Design review of the part built by this model. Coordinates are the model's own, in mm. A direction names the side the tool comes from. Coordinates: 2 decimals unless noted, no trailing zeros. Write each loop counter-clockwise with the first axis right and the second up, starting at its lowest first coordinate (ties: lowest second). Pieces come first, ordered by that corner, then holes.
Q1. To check wall thickness, follow probe 1 along Z at (x, y) = (17, 17); probe 2 along Y at (x, z) = (93.5, 8.5); probe 3 along Y at (x, z) = (9.5, 7). State the ranges of each line that lie inside material, in increasing order.
Q2. Add section B-B, the plane x = 29. Give the boundary of the cut face in (y, z).
Q3. The part is to be moulded in two halves that separate along Z. For faces 4 (the face through (49, 20.802, 8)), 5 (the face through (50.7, -7.28, 16.28)), 6 (the face through (50.65, -9.83, 13.26)), 7 (the face through (50.651, 15.738, 7.519)), say which applies: +Z half, -Z half, draft (parallel to the pull), parting line (faces both ways), or undercut.
Q4. Machinability: for faces 1 (the face through (49, 19, 10.229)), 2 (the face through (98, -7, 15.073)), 3 (the face through (2, -7, 15.073)), which of the approach directions +Z, -Z, +X, -X, +Y, -Y give a long, thin tool a straight path to every point of the face, cutting with its end or side? Answer none if there is none.
Q5. Clearance check with flat-ended pins moving along their axes: pin 1 Ø8 at (y, z) = (0.5, 9) entering from -X; pin 2 Ø4 at (y, z) = (16.8, 8.07) entering from +X; pin 3 Ø2 at (x, z) = (34.5, 18) entering from +Y; pin 4 Ø5 at (y, z) = (-5.5, 18.5) entering from -X. State where each tip first meets the part, or that it passes through.
Q6. Add section A-A, the plane y = 19.5. Give the boundary of the cut face in (x, z).
Q7. Add section C-C, the plane z = 18.5. Give the boundary of the cut face in (x, y).
from build123d import *

# Parameters (mm, degrees)
SKETCH1_W           = 14
SKETCH1_H           = 27
BOSS_EXTRUDE1_DEPTH = 100
CUT_EXTRUDE1_DEPTH  = 100
FILLET1_R           = 10
SKETCH4_W           = 98.852101938
SKETCH4_H           = 4.155908349
BOSS_EXTRUDE2_DEPTH = 4
SKETCH5_R           = 1.2
SKETCH5_R_2         = 0.6
CUT_EXTRUDE2_DEPTH  = 100
CHAMFER1_SIZE       = 7
SKETCH6_W           = 4.155908349
SKETCH6_H           = 24
CUT_EXTRUDE3_DEPTH  = 3.5
SKETCH8_W           = 1.147898062
SKETCH8_H           = 4.155908349
BOSS_EXTRUDE3_DEPTH = 4
SKETCH9_W           = 4.155908349
SKETCH9_H           = 24
CUT_EXTRUDE4_DEPTH  = 3.5
SKETCH10_W          = 10.233519384
SKETCH10_H          = 31.339386183
CUT_EXTRUDE5_DEPTH  = 3.5
SKETCH11_W          = 18.924548437
SKETCH11_H          = 36.127134787
CUT_EXTRUDE7_DEPTH  = 3.5
FILLET2_R           = 5
FILLET5_R           = 1
FILLET6_R           = 1


with BuildPart() as part:
    # Sketch1 → Boss-Extrude1 (new body)
    with BuildSketch(Plane(origin=(0, 0, 0), x_dir=(0, 0, -1), z_dir=(1, 0, 0))):
        with Locations((-13.07263952, 3.302202671)):
            Rectangle(SKETCH1_W, SKETCH1_H)
    extrude(amount=BOSS_EXTRUDE1_DEPTH)

    # Sketch2 → Cut-Extrude1 (cut)
    with BuildSketch(Plane(origin=(100, 0, 0), x_dir=(0, 0, -1), z_dir=(1, 0, 0))):
        Polygon((-20.07263952, -10.197797329), (-15.511656896, -8.952001224), (-10.228547869, 16.802202671), (-20.07263952, 16.802202671), align=None)
    extrude(amount=-CUT_EXTRUDE1_DEPTH, mode=Mode.SUBTRACT)

    # Fillet1
    # the kernel refuses this fillet: 10 mm, written as the material it adds along each edge
    with BuildSketch(Plane(origin=(100, -8.952001224, 15.511656896), x_dir=(0, 0.9796012375346099, -0.20095127623546138), z_dir=(-1, 0, 0))) as fillet1_piece_1_section:
        with BuildLine():
            CenterArc((6.021748433, -10), FILLET1_R, 90, 54.673150745)
            Line((-2.136918685, -4.217599905), (-2.300092028, -4.101951904))
            ThreePointArc((-2.300092028, -4.101951904), (-1.246866474, -2.018406947), (-0.178407131, 0.090393006))
            Line((-0.178407131, 0.090393006), (0, 0.2))
            Line((0, 0.2), (6.021748433, 0.2))
            Line((6.021748433, 0.2), (6.021748433, 0))
        make_face()
    fillet1_piece_1 = extrude(amount=100, mode=Mode.PRIVATE)
    fillet1_piece_1 = split(fillet1_piece_1, bisect_by=Plane(origin=(50, -10.197797329, 16.270514602), z_dir=(0, 1, 0)), keep=Keep.TOP, mode=Mode.PRIVATE)
    add(fillet1_piece_1)

    # Sketch4 → Boss-Extrude2 (add)
    with BuildSketch(Plane(origin=(0, 16.802202671, 0), x_dir=(1, 0, 0), z_dir=(0, 1, 0))):
        with Locations((50.573949031, -8.150593694)):
            Rectangle(SKETCH4_W, SKETCH4_H)
    extrude(amount=BOSS_EXTRUDE2_DEPTH)

    # Sketch5 → Cut-Extrude2 (cut)
    with BuildSketch(Plane(origin=(100, 0, 0), x_dir=(0, 0, -1), z_dir=(1, 0, 0))):
        with Locations((-8.07263952, 16.802202671)):
            Circle(SKETCH5_R)
        with Locations((-8.07263952, -1.197797329)):
            Circle(SKETCH5_R_2)
    extrude(amount=-CUT_EXTRUDE2_DEPTH, mode=Mode.SUBTRACT)

    # Chamfer1
    chamfer1_edges = [part.edges().sort_by_distance(p)[0] for p in [
        (50, -10.197797329, 6.07263952),
    ]]
    chamfer(chamfer1_edges, length=CHAMFER1_SIZE)

    # Sketch6 → Cut-Extrude3 (cut)
    with BuildSketch(Plane(origin=(100, 0, 0), x_dir=(0, 0, -1), z_dir=(1, 0, 0))):
        with Locations((-8.150593694, 8.802202671)):
            Rectangle(SKETCH6_W, SKETCH6_H)
    extrude(amount=-CUT_EXTRUDE3_DEPTH, mode=Mode.SUBTRACT)

    # Sketch8 → Boss-Extrude3 (add)
    with BuildSketch(Plane(origin=(0, 16.802202671, 0), x_dir=(1, 0, 0), z_dir=(0, 1, 0))):
        with Locations((0.573949031, -8.150593694)):
            Rectangle(SKETCH8_W, SKETCH8_H)
    extrude(amount=BOSS_EXTRUDE3_DEPTH)

    # Sketch9 → Cut-Extrude4 (cut)
    with BuildSketch(Plane.ZY):
        with Locations((8.150593694, 8.802202671)):
            Rectangle(SKETCH9_W, SKETCH9_H)
    extrude(amount=-CUT_EXTRUDE4_DEPTH, mode=Mode.SUBTRACT)

    # Sketch10 → Cut-Extrude5 (cut)
    with BuildSketch(Plane.ZY):
        with Locations((9.955879828, 5.471895763)):
            Rectangle(SKETCH10_W, SKETCH10_H)
    extrude(amount=-CUT_EXTRUDE5_DEPTH, mode=Mode.SUBTRACT)

    # Sketch11 → Cut-Extrude7 (cut)
    with BuildSketch(Plane(origin=(100, 0, 0), x_dir=(0, 0, -1), z_dir=(1, 0, 0))):
        with Locations((-5.610365301, 7.865770065)):
            Rectangle(SKETCH11_W, SKETCH11_H)
    extrude(amount=-CUT_EXTRUDE7_DEPTH, mode=Mode.SUBTRACT)

    # Fillet2
    fillet2_edges = [part.edges().sort_by_distance(p)[0] for p in [
        (50, -10.197797329, 13.07263952),
    ]]
    fillet(fillet2_edges, radius=FILLET2_R)

    # Fillet5
    # the kernel refuses this fillet: 1 mm, written as the material it takes off along each edge
    with BuildSketch(Plane(origin=(102.500000319, -10.19729224, 15.07263952), x_dir=(0, -0.0005050888353824425, 0.9999998724426261), z_dir=(-1, 0, 0))) as fillet5_piece_1:
        with BuildLine():
            CenterArc((0.999495039, 0.999999872), FILLET5_R, 180.02893946, 90)
            Line((-0.000504834, 0.999494784), (-0.100504821, 0.999444275))
            Line((-0.100504821, 0.999444275), (-0.099999987, -5.0509e-05))
            Line((-0.099999987, -5.0509e-05), (-0.001370852, -0.099990603))
            ThreePointArc((-0.001370852, -0.099990603), (0.071118567, -0.100469181), (1.000050636, -0.099999987))
            Line((1.000050636, -0.099999987), (1.000000128, 0))
        make_face()
    extrude(amount=6.000000319, mode=Mode.SUBTRACT)

    # Fillet6
    # the kernel refuses this fillet: 1 mm, written as the material it takes off along each edge
    with BuildSketch(Plane(origin=(-2.500000319, -10.19729224, 15.07263952), x_dir=(0, 1, 0), z_dir=(1, 0, 0))) as fillet6_piece_1:
        with BuildLine():
            CenterArc((0.999494911, 1), FILLET6_R, 180, 90)
            Line((-0.000505089, 1), (-0.100505089, 1))
            ThreePointArc((-0.100505089, 1), (-0.100505089, 0.071067812), (-0.099989898, -0.001421356))
            Line((-0.099989898, -0.001421356), (0, -0.1))
            Line((0, -0.1), (0.999494911, -0.1))
            Line((0.999494911, -0.1), (0.999494911, 0))
        make_face()
    extrude(amount=6.000000319, mode=Mode.SUBTRACT)


solid = part.part
Here are the results:
1. probe 1: z = 6.07 to 6.89, 9.26 to 10.23
1. probe 2: y = -5.63 to -1.62, -0.78 to 15.68, 17.92 to 20.8
1. probe 3: y = -4.13 to 16.26, 17.34 to 20.8
2. outline: (-10.2, 15.14) arc R5 ccw to (-8.73, 11.61) - (-3.2, 6.07) - (20.8, 6.07) - (20.8, 10.23) - (16.8, 10.23) - (-3.05, 14.3) arc R10 cw to (-10.2, 20.07) - close; hole circle Ø1.2 at (-1.2, 8.07); hole circle Ø2.4 at (16.8, 8.07)
3. face 4: draft
3. face 5: +Z half
3. face 6: -Z half
3. face 7: undercut
4. face 1: +Z, +X, -X, +Y
4. face 2: -Z, +X, +Y, -Y
4. face 3: -Z, -X, +Y, -Y
5. pin 1: stops at x = 3.5
5. pin 2: stops at x = 96.5
5. pin 3: stops at y = -8.09
5. pin 4: passes through
6. outline: (3.5, 6.07) - (96.5, 6.07) - (96.5, 10.23) - (3.5, 10.23) - close
7. outline: (0, -10.2) - (100, -10.2) - (100, -9.33) - (0, -9.33) - close
